```python
from build123d import *

# Parameters (mm, degrees)
SKETCH_1_W                   = 20
SKETCH_1_H                   = 20
EXTRUDE_1_DEPTH              = 10
HOLE_WIZARD_M3_2_D           = 2.5
HOLE_WIZARD_M3_2_DEPTH       = 5
HOLE_WIZARD_M3_2_TIP         = 0.751075774
HOLE_WIZARD_M3_3_D           = 2.5
HOLE_WIZARD_M3_3_DEPTH       = 6
HOLE_WIZARD_M3_3_CSINK_D     = 3.05
HOLE_WIZARD_M3_3_CSINK_ANGLE = 90
HOLE_WIZARD_M3_3_TIP         = 1.25
SKETCH_23_R                  = 2.5
CUT_EXTRUDE_1_DEPTH          = 11
SKETCH_40_R                  = 1
CUT_EXTRUDE_2_DEPTH          = 3


with BuildPart() as part:
    # 草图1 → 凸台-拉伸1 (new body)
    with BuildSketch(Plane(origin=(0, 0, 0), x_dir=(1, 0, 0), z_dir=(0, 1, 0))):
        Rectangle(SKETCH_1_W, SKETCH_1_H)
    extrude(amount=EXTRUDE_1_DEPTH)

    # 草图26 → Ø6.1 (6.1) 直径孔1 (revolve, cut)
    with BuildSketch(Plane(origin=(5.3, 5, 10), x_dir=(0, -1, 0), z_dir=(1, 0, 0))):
        Polygon((0, 0), (0, 20), (3.3, 20), (3.05, 19.75), (3.05, 0.25), (3.3, 0), align=None)
    revolve(axis=Axis((5.3, 5, 16.35), (0, 0, -1)), mode=Mode.SUBTRACT)

    # M3 螺纹孔2
    with Locations(Plane.XY.offset(10)):
        with Locations((-1.5, 5)):
            Hole(HOLE_WIZARD_M3_2_D / 2, depth=HOLE_WIZARD_M3_2_DEPTH)
            with Locations((0, 0, -(HOLE_WIZARD_M3_2_DEPTH + HOLE_WIZARD_M3_2_TIP / 2))):  # 118° drill point
                Cone(0, HOLE_WIZARD_M3_2_D / 2, HOLE_WIZARD_M3_2_TIP, mode=Mode.SUBTRACT)

    # M3 螺纹孔3
    with Locations(Plane(origin=(0, 10, 0), x_dir=(1, 0, 0), z_dir=(0, 1, 0))):
        with Locations((5.3, 0)):
            CounterSinkHole(HOLE_WIZARD_M3_3_D / 2, HOLE_WIZARD_M3_3_CSINK_D / 2, depth=HOLE_WIZARD_M3_3_DEPTH, counter_sink_angle=HOLE_WIZARD_M3_3_CSINK_ANGLE)
            with Locations((0, 0, -(HOLE_WIZARD_M3_3_DEPTH + HOLE_WIZARD_M3_3_TIP / 2))):  # 90° drill point
                Cone(0, HOLE_WIZARD_M3_3_D / 2, HOLE_WIZARD_M3_3_TIP, mode=Mode.SUBTRACT)

    # 草图23 → 切除-拉伸1 (cut, through all)
    with BuildSketch(Plane(origin=(0, 10, 0), x_dir=(1, 0, 0), z_dir=(0, 1, 0))):
        with Locations((-4.3, 0)):
            Circle(SKETCH_23_R)
    extrude(amount=-CUT_EXTRUDE_1_DEPTH, mode=Mode.SUBTRACT)

    # 草图40 → 切除-拉伸2 (cut)
    with BuildSketch(Plane.XY.offset(10)):
        with Locations((-1.1, 8.4)):
            Circle(SKETCH_40_R)
    extrude(amount=-CUT_EXTRUDE_2_DEPTH, mode=Mode.SUBTRACT)


solid = part.part
```
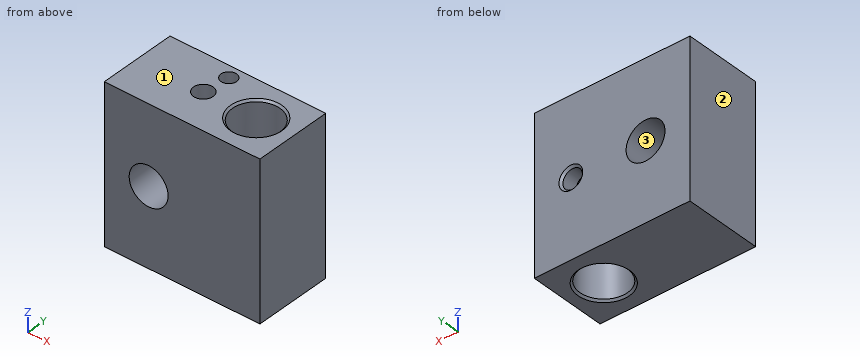
Can you work these out from the model? Positions are in its coordinate system, mm. Face numbers are marked on the shaded views. Round coordinates to 2 decimals unless told otherwise and drop trailing zeros. Loops run counter-clockwise (first coordinate to the right, second up) from the corner with the lowest first, then second, coordinate; pieces in that order, holes last.
Item 1: Suppose I cut it at D-D, the plane z = 3.25. Write out the boundary of the cut face in (x, y).
Item 2: Suppose I cut it at A-A, the plane x = 5.3. Write out the boundary of the cut face in (y, z) (3 decimals).
Item 3: If we mould it in two halves opening along Z, with no side actions, what happens to the marked faces 1, 2 and 3? For each: +Z half, -Z half, draft (parallel to the pull), parting line (faces both ways), or undercut.
Item 4: Suppose I cut it at B-B, the plane z = 0. Write out the boundary of the cut face in (x, y) (3 decimals).
Item 5: Will these pins go through, and if not, where does the flat tip stop? pin 1 Ø8 at (x, z) = (-4.3, 0) entering from -Y; pin 2 Ø1 at (x, y) = (-1, 8) entering from +Z.
Item 6: Please list where these lines run through material, in increasing order: L1, parallel to X at y = 5, z = 7.3; L2, parallel to Y at x = -1.5, z = 8.6; L3, parallel to Y at x = -1.1, z = 8.5.
Item 7: Suppose I cut it at C-C, the plane y = 1. Write out the boundary of the cut face in (x, z).
Reported:
1. outline: (-10, 0) - (10, 0) - (10, 10) - (-10, 10) - close; hole circle Ø6.1 at (5.3, 5)
2. outline: (0, -10) - (1.7, -10) - (1.95, -9.75) - (1.95, 9.75) - (1.7, 10) - (0, 10) - close; (8.05, -9.75) - (8.3, -10) - (10, -10) - (10, -1.525) - (9.725, -1.25) - (8.05, -1.25) - close; (8.05, 1.25) - (9.725, 1.25) - (10, 1.525) - (10, 10) - (8.3, 10) - (8.05, 9.75) - close
3. face 1: +Z half
3. face 2: draft
3. face 3: undercut
4. outline: (-10, 0) - (-6.8, 0) - (-6.8, 10) - (-10, 10) - close; (-1.8, 0) - (10, 0) - (10, 10) - (6.825, 10) - (6.55, 9.725) - (6.55, 7.782) arc R3.05 cw (long way) to (4.05, 7.782) - (4.05, 9.725) - (3.775, 10) - (-1.8, 10) - close
5. pin 1: stops at y = 0
5. pin 2: stops at z = 7
6. L1: x = -10 to -2.75, -0.25 to 2.25, 8.35 to 10
6. L2: y = 0 to 3.75, 6.25 to 7.48, 9.32 to 10
6. L3: y = 0 to 3.82, 6.18 to 7.4, 9.4 to 10
7. outline: (-10, -10) - (10, -10) - (10, 10) - (-10, 10) - close; hole circle Ø5 at (-4.3, 0)
